Part print with two shaded views. Sizes in mm from the minimum x, y, z corner. A direction names the side the tool comes from. Round coordinates to 2 decimals unless told otherwise and drop trailing zeros. Write each loop counter-clockwise with the first axis right and the second up, starting at its lowest first coordinate (ties: lowest second). Pieces come first, ordered by that corner, then holes. Notation, with made-up numbers: (85.25, 85) -> (107.25, 85) arc R26 ccw to (107.25, 123) -> close; hole circle Ø4 at (77.25, 36). An arc over 180 degrees is marked (long way). Answer in a Markdown table with one row per item. Add a question column.
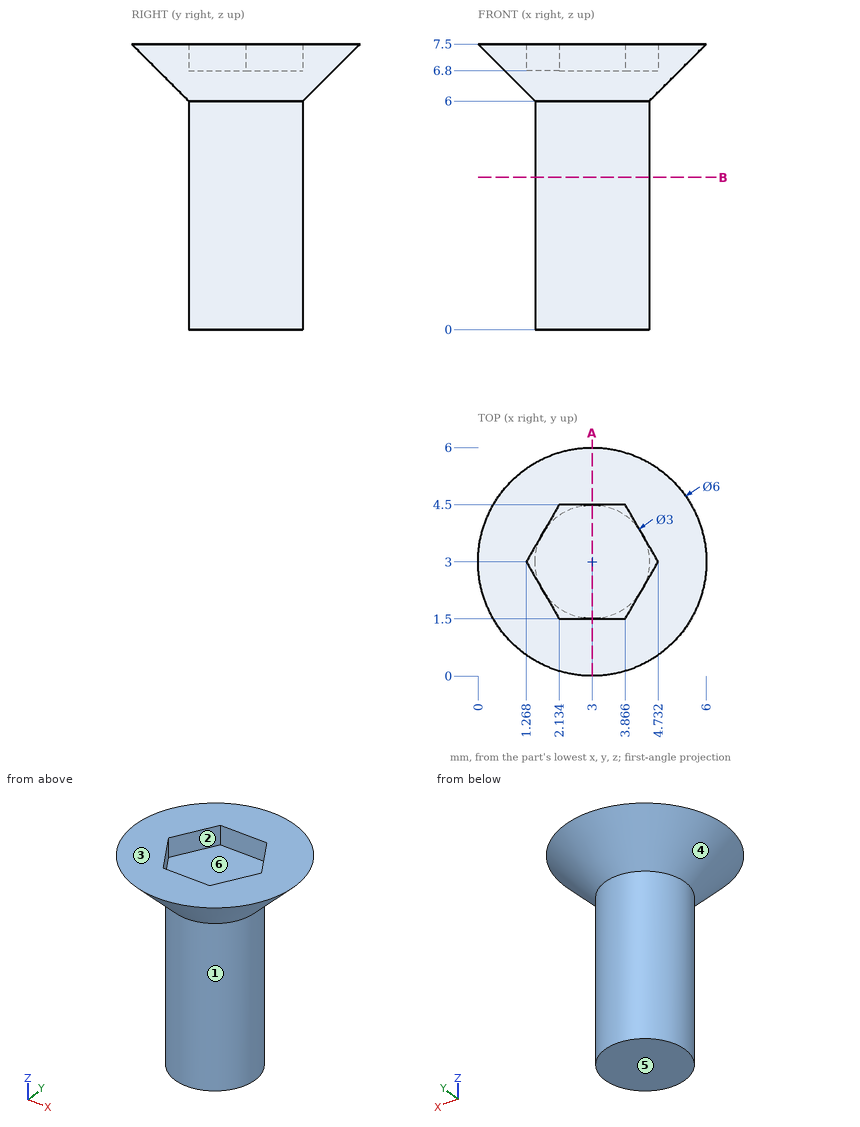
Item 1: Pin check, flat tips, straight feed: pin 1 (1 mm diameter, centred on x = 4, z = 5.5, fed in from -Y); pin 2 (3 mm diameter, centred on x = 3.5, y = 4, fed in from -Z); pin 3 (1.5 mm diameter, centred on x = 4.5, z = 3, fed in from +Y); pin 4 (0.6 mm diameter, centred on x = 3, z = 7, fed in from +Y). Stop position of each tip, or through.
Item 2: Saw through at B-B on z = 4. Give the cut face in (x, y), then the cut area to 3 significant figures.
Item 3: Saw through at A-A on x = 3. Give the cut face in (y, z), then the cut area to 4 significant figures.
Item 4: Tool access for the marked faces 1, 2 and 3: list every direction of +Z, -Z, +X, -X, +Y, -Y with a clear straight run to the whole face (end or side of a thin tool).
Item 5: Drill centre lines: probe 1 along Z at (x, y) = (3.55, 3.05); probe 2 along Y at (x, z) = (2.95, 5.75); probe 3 along X at (y, z) = (2.75, 6.5). Where is each one in solid material? Low to high.
Item 6: Two-plate mould, pull along X, no slides. Class the marked faces 4, 5 and 6: +X half, -X half, draft (parallel to the pull), parting line (faces both ways), or undercut.
Recorded:
| question | item | result |
|---|---|---|
| 1 | pin 1 | y = 1.59 |
| 1 | pin 2 | z = 0 |
| 1 | pin 3 | y = 4.3 |
| 1 | pin 4 | y = 5.8 |
| 2 | outline | circle Ø3 at (3, 3) |
| 2 | area | 7.07 mm2 |
| 3 | outline | (0, 7.5) -> (1.5, 6) -> (1.5, 0) -> (4.5, 0) -> (4.5, 6) -> (6, 7.5) -> (4.5, 7.5) -> (4.5, 6.8) -> (1.5, 6.8) -> (1.5, 7.5) -> close |
| 3 | area | 22.65 mm2 |
| 4 | face 1 | -Z |
| 4 | face 2 | +Z |
| 4 | face 3 | +Z, +X, -X, +Y, -Y |
| 5 | probe 1 | 0 to 6.8 |
| 5 | probe 2 | 1.5 to 4.5 |
| 5 | probe 3 | 1.02 to 4.98 |
| 6 | face 4 | parting line |
| 6 | face 5 | draft |
| 6 | face 6 | undercut |
